The model under review builds one solid part; all positions refer to its coordinate system, in mm. A direction names the side the tool comes from. Give positions to 0.01 mm unless a question says otherwise; leave off trailing zeros. Loops run counter-clockwise (first coordinate to the right, second up) from the corner with the lowest first, then second, coordinate; pieces in that order, holes last. Notation, with made-up numbers: (28.25, 33.25) - (81.25, 33.25) arc R7 cw to (81.25, 44.25) - close; hole circle Ø10 at (79, 82.5). An arc over 180 degrees is marked (long way). Answer as a JSON object with one key per item and string values.
from build123d import *

# Parameters (mm, degrees)
BOSS_EXTRUDE3_DEPTH = 14
SKETCH3_R           = 4.84
CUT_EXTRUDE3_DEPTH  = 14.0462
CUT_EXTRUDE4_DEPTH  = 3
MIRROR1_START       = 11
MIRROR1_DEPTH       = 3
MIRROR1_2_DEPTH     = 11
MIRROR1_3_DEPTH     = 3
SKETCH6_W           = 32.77755098
SKETCH6_H           = 97.199429117
CUT_EXTRUDE6_DEPTH  = 68.951679292
FILLET1_R           = 10
FILLET2_R           = 10
FILLET3_R           = 10
FILLET4_R           = 10


# Read off the part's stored shape, not the designer's step: Mirror1
with BuildPart() as part:
    # Sketch1 → Boss-Extrude3 (new body)
    with BuildSketch(Plane.YZ):
        with BuildLine():
            Line((-28.968617751, -12.789334175), (28.968617751, -12.789334175))
            ThreePointArc((28.968617751, -12.789334175), (44.579120821, 0), (35.110840206, 17.821518929))
            ThreePointArc((35.110840206, 17.821518929), (30.644623053, 21.505675602), (28.968617751, 27.047436358))
            Line((28.968617751, 27.047436358), (28.968617751, 39.053986921))
            ThreePointArc((28.968617751, 39.053986921), (26.039685563, 46.125054733), (18.968617751, 49.053986921))
            Line((18.968617751, 49.053986921), (-18.968617751, 49.053986921))
            ThreePointArc((-18.968617751, 49.053986921), (-26.039685563, 46.125054733), (-28.968617751, 39.053986921))
            Line((-28.968617751, 39.053986921), (-28.968617751, 27.047436358))
            ThreePointArc((-28.968617751, 27.047436358), (-30.644623053, 21.505675602), (-35.110840206, 17.821518929))
            ThreePointArc((-35.110840206, 17.821518929), (-44.579120821, 0), (-28.968617751, -12.789334175))
        make_face()
    extrude(amount=BOSS_EXTRUDE3_DEPTH)

    # Sketch3 → Cut-Extrude3 (cut)
    with BuildSketch(Plane.YZ.offset(14)):
        with Locations(Location((0, 3.132326373, 0), (0, 0, 270))):
            Circle(SKETCH3_R)
    extrude(amount=-CUT_EXTRUDE3_DEPTH, mode=Mode.SUBTRACT)

    # Sketch4 → Cut-Extrude4 (cut)
    with BuildSketch(Plane.YZ.offset(14)):
        with BuildLine():
            Line((-12.95, 49.053986921), (-12.95, 31.267703884))
            ThreePointArc((-12.95, 31.267703884), (0, 18.317703884), (12.95, 31.267703884))
            Line((12.95, 31.267703884), (12.95, 49.053986921))
            Line((12.95, 49.053986921), (-12.95, 49.053986921))
        make_face()
    extrude(amount=-CUT_EXTRUDE4_DEPTH, mode=Mode.SUBTRACT)

    # Mirror1 outline → Mirror1 (cut)
    with BuildSketch(Plane.YZ.offset(MIRROR1_START)):
        with BuildLine():
            ThreePointArc((4.30437196, -12.789334175), (0, -12.053051137), (-4.30437196, -12.789334175))
            Line((-4.30437196, -12.789334175), (4.30437196, -12.789334175))
        make_face()
    extrude(amount=MIRROR1_DEPTH, mode=Mode.SUBTRACT)

    # Mirror1 2 outline → Mirror1 2 (add)
    with BuildSketch(Plane.YZ):
        with BuildLine():
            ThreePointArc((-28.968617751, -32.789334175), (-26.039685563, -39.860401987), (-18.968617751, -42.789334175))
            Line((-18.968617751, -42.789334175), (18.968617751, -42.789334175))
            ThreePointArc((18.968617751, -42.789334175), (26.039685563, -39.860401987), (28.968617751, -32.789334175))
            Line((28.968617751, -32.789334175), (28.968617751, -20.782783611))
            ThreePointArc((28.968617751, -20.782783611), (30.644623053, -15.241022855), (35.110840206, -11.556866182))
            ThreePointArc((35.110840206, -11.556866182), (32.100944124, -12.478176697), (28.968617751, -12.789334175))
            Line((28.968617751, -12.789334175), (-28.968617751, -12.789334175))
            ThreePointArc((-28.968617751, -12.789334175), (-32.100944124, -12.478176697), (-35.110840206, -11.556866182))
            ThreePointArc((-35.110840206, -11.556866182), (-30.644623053, -15.241022855), (-28.968617751, -20.782783611))
            Line((-28.968617751, -20.782783611), (-28.968617751, -32.789334175))
        make_face()
    extrude(amount=MIRROR1_2_DEPTH)

    # Mirror1 3 outline → Mirror1 3 (add)
    with BuildSketch(Plane.YZ.offset(MIRROR1_START)):
        with BuildLine():
            ThreePointArc((-28.968617751, -32.789334175), (-26.039685563, -39.860401987), (-18.968617751, -42.789334175))
            Line((-18.968617751, -42.789334175), (-12.95, -42.789334175))
            Line((-12.95, -42.789334175), (-12.95, -25.003051137))
            ThreePointArc((-12.95, -25.003051137), (-10.569865583, -17.521043281), (-4.30437196, -12.789334175))
            Line((-4.30437196, -12.789334175), (-28.968617751, -12.789334175))
            ThreePointArc((-28.968617751, -12.789334175), (-32.100944124, -12.478176697), (-35.110840206, -11.556866182))
            ThreePointArc((-35.110840206, -11.556866182), (-30.644623053, -15.241022855), (-28.968617751, -20.782783611))
            Line((-28.968617751, -20.782783611), (-28.968617751, -32.789334175))
        make_face()
        with BuildLine():
            Line((12.95, -25.003051137), (12.95, -42.789334175))
            Line((12.95, -42.789334175), (18.968617751, -42.789334175))
            ThreePointArc((18.968617751, -42.789334175), (26.039685563, -39.860401987), (28.968617751, -32.789334175))
            Line((28.968617751, -32.789334175), (28.968617751, -20.782783611))
            ThreePointArc((28.968617751, -20.782783611), (30.644623053, -15.241022855), (35.110840206, -11.556866182))
            ThreePointArc((35.110840206, -11.556866182), (32.100944124, -12.478176697), (28.968617751, -12.789334175))
            Line((28.968617751, -12.789334175), (4.30437196, -12.789334175))
            ThreePointArc((4.30437196, -12.789334175), (10.569865583, -17.521043281), (12.95, -25.003051137))
        make_face()
        with BuildLine():
            ThreePointArc((-4.304371959, 19.053986921), (0, 18.317703884), (4.304371959, 19.053986921))
            Line((4.304371959, 19.053986921), (-4.304371959, 19.053986921))
        make_face()
    extrude(amount=MIRROR1_3_DEPTH)

    # Sketch6 → Cut-Extrude6 (cut, through all)
    with BuildSketch(Plane.YZ.offset(14)):
        with Locations((-32.348084365, 0.454272362)):
            Rectangle(SKETCH6_W, SKETCH6_H)
        with Locations((32.348084365, 0.454272362)):
            Rectangle(SKETCH6_W, SKETCH6_H)
    extrude(amount=-CUT_EXTRUDE6_DEPTH, mode=Mode.SUBTRACT)

    # Fillet1
    fillet1_edges = [part.edges().sort_by_distance(p)[0] for p in [
        (0, -15.959308875, 3.132326373),
    ]]
    fillet(fillet1_edges, radius=FILLET1_R)

    # Fillet2
    fillet2_edges = [part.edges().sort_by_distance(p)[0] for p in [
        (0, 5, -42.789334175),
        (2.928932188, -13.030376687, -42.789334175),
        (12, -15.959308875, -42.789334175),
    ]]
    fillet(fillet2_edges, radius=FILLET2_R)

    # Fillet3
    fillet3_edges = [part.edges().sort_by_distance(p)[0] for p in [
        (0, 5, 49.053986921),
        (2.928932188, -13.030376687, 49.053986921),
        (12, -15.959308875, 49.053986921),
    ]]
    fillet(fillet3_edges, radius=FILLET3_R)

    # Fillet4
    fillet4_edges = [part.edges().sort_by_distance(p)[0] for p in [
        (12, 15.959308875, -42.789334175),
        (2.928932188, 15.959308875, -39.860401987),
        (0, 15.959308875, 3.132326373),
        (2.928932188, 15.959308875, 46.125054733),
        (12, 15.959308875, 49.053986921),
    ]]
    fillet(fillet4_edges, radius=FILLET4_R)


solid = part.part
Q1. To check wall thickness, follow probe 1 along Y at (x, z) = (13.25, -27); probe 2 along Y at (x, z) = (9.75, -7); probe 3 along X at (y, z) = (-6.5, -15.5). State the ranges of each line that lie inside material, in increasing order. Write a range as [from, to].
Results:
{"probe 1": "y = [-15.96, -12.95], [12.95, 15.96]", "probe 2": "y = [-15.96, 15.96]", "probe 3": "x = [0.01, 11]"}
Q2. The part is to be moulded in two halves that separate along Y. For faces 4 (the face through (0, -5, 4)), 5 (the face through (12, 15.959, 3)), 6 (the face through (12, -12.95, -33)), 7 (the face through (3, -13.1, 3.6)), say which applies: +Y half, -Y half, draft (parallel to the pull), parting line (faces both ways), or undercut.
Results:
{"face 4": "draft", "face 5": "+Y half", "face 6": "undercut", "face 7": "-Y half"}
Q3. Consider section B-B, the plane z = 5. State the section outline as (x, y) points, plus the area to 3 significant figures.
Results:
{"outline": "(0, -5.96) arc R10 ccw to (10, -15.96) - (14, -15.96) - (14, -4.47) - (0, -4.47) - close; (0, 4.47) - (14, 4.47) - (14, 15.96) - (10, 15.96) arc R10 ccw to (0, 5.96) - close", "area": "279 mm^2"}
Q4. Consider section C-C, the plane x = 8.25. State the section outline as (y, z) points (3 decimals), plus the area to 3 significant figures.
Results:
{"outline": "(-15.805, -32.789) arc R9.846 ccw to (-5.959, -42.635) - (5.959, -42.635) arc R9.846 ccw to (15.805, -32.789) - (15.805, 39.054) arc R9.846 ccw to (5.959, 48.9) - (-5.959, 48.9) arc R9.846 ccw to (-15.805, 39.054) - close; hole circle Ø9.68 at (0, 3.132)", "area": "2,740 mm^2"}
Q5. For faces 1 (the face through (3.01, 0.08, -39.94)), 2 (the face through (11, 0, -27)), 3 (the face through (11, 0, 34)), list the 3-axis set-ups (+Z, -Z, +X, -X, +Y, -Y) from which the entire face can be reached by the end or side of a thin tool; tool diameter is ignored.
Results:
{"face 1": "-Z, -X, +Y, -Y", "face 2": "-Z, +X", "face 3": "+Z, +X"}
Q6. Clearance check with flat-ended pins moving along their axes: pin 1 Ø6 at (y, z) = (0, 3.13) entering from -X; pin 2 Ø6 at (x, z) = (2.5, 23.5) entering from +Y; pin 3 Ø4 at (x, z) = (7, 13.5) entering from +Y; pin 4 Ø0.9 at (x, z) = (13, -33.5) entering from +Y. State where each tip first meets the part, or that it passes through.
Results:
{"pin 1": "passes through", "pin 2": "stops at y = 14.89", "pin 3": "stops at y = 15.91", "pin 4": "stops at y = 15.96"}
Q7. Consider section D-D, the plane z = -22.5. State the section outline as (x, y) points.
Results:
{"outline": "(0, -5.96) arc R10 ccw to (10, -15.96) - (14, -15.96) - (14, -12.71) - (11, -12.71) - (11, 12.71) - (14, 12.71) - (14, 15.96) - (10, 15.96) arc R10 ccw to (0, 5.96) - close"}
Q8. Consider section A-A, the plane y = 0. State the section outline as (x, z) points.
Results:
{"outline": "(0, -32.79) arc R10 ccw to (10, -42.79) - (11, -42.79) - (11, -12.05) - (14, -12.05) - (14, -1.71) - (0, -1.71) - close; (0, 7.97) - (14, 7.97) - (14, 19.05) - (11, 19.05) - (11, 49.05) - (10, 49.05) arc R10 ccw to (0, 39.05) - close"}
